For this review, take the finished solid that the model builds, in its own axes (mm). Face numbers are marked on the shaded views. Round coordinates to 2 decimals unless told otherwise and drop trailing zeros. Order: outer loops, then holes, each group sorted by start corner. A loop starts at its lowest first (then second) coordinate and runs counter-clockwise, first axis right, second up. Notation, with made-up numbers: M -35,55.25 L -18,55.25 A17 ccw -18,73.25 Z; hole C 10.5,-13.75 d5. An arc over 180 degrees is marked long. Use a Markdown table: item, result.
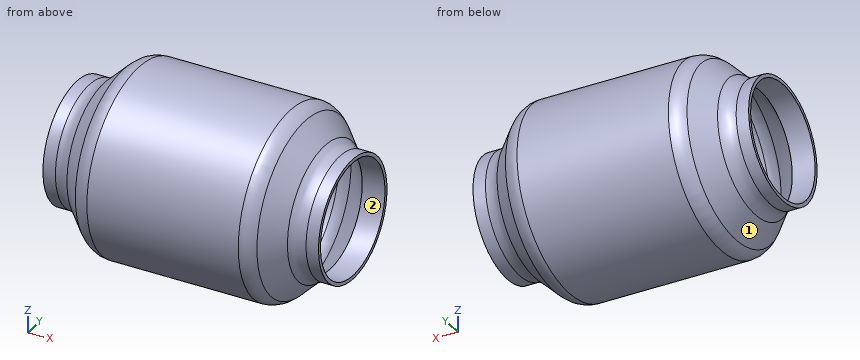
from build123d import *


with BuildPart() as part:
    # Sketch1 → Revolve1 (revolve)
    with BuildSketch(Plane.XY):
        with BuildLine():
            Line((-123.19, 53.975), (-123.19, 50.8))
            Line((-123.19, 50.8), (-102.824871939, 50.8))
            Line((-102.824871939, 50.8), (-79.829487758, 73.795384182))
            ThreePointArc((-79.829487758, 73.795384182), (-73.649222963, 77.924905094), (-66.359103576, 79.375))
            Line((-66.359103576, 79.375), (66.359103576, 79.375))
            ThreePointArc((66.359103576, 79.375), (73.649222963, 77.924905094), (79.829487758, 73.795384182))
            Line((79.829487758, 73.795384182), (102.824871939, 50.8))
            Line((102.824871939, 50.8), (123.19, 50.8))
            Line((123.19, 50.8), (123.19, 53.975))
            Line((123.19, 53.975), (112.030768363, 53.975))
            ThreePointArc((112.030768363, 53.975), (104.740648977, 55.425094906), (98.560384182, 59.554615818))
            Line((98.560384182, 59.554615818), (81.144615818, 76.970384182))
            ThreePointArc((81.144615818, 76.970384182), (74.964351023, 81.099905094), (67.674231637, 82.55))
            Line((67.674231637, 82.55), (-67.674231637, 82.55))
            ThreePointArc((-67.674231637, 82.55), (-74.964351023, 81.099905094), (-81.144615818, 76.970384182))
            Line((-81.144615818, 76.970384182), (-98.560384182, 59.554615818))
            ThreePointArc((-98.560384182, 59.554615818), (-104.740648977, 55.425094906), (-112.030768363, 53.975))
            Line((-112.030768363, 53.975), (-123.19, 53.975))
        make_face()
    revolve(axis=Axis((-123.19, 0, 0), (1, 0, 0)))


solid = part.part
Q1. Add section A-A (x = 11). Write out the cut boundary in (y, z) (3 decimals), then the cut area to 3 significant figures.
Determined:
| item | result |
|---|---|
| outline | C 0,0 d165.1; hole C 0,0 d158.75 |
| area | 1,620 mm^2 |
Q2. Wall thickness on line 1 along Z through (x, y) = (-27, 0) (3 decimals); line 2 along X through (y, z) = (12.5, 58.5); line 3 along Y through (x, z) = (-89, 15.5): over which ranges is each line inside the solid? List them lowest first. Write a range as [from, to].
Determined:
| item | result |
|---|---|
| line 1 | z = [-82.55, -79.375], [79.375, 82.55] |
| line 2 | x = [-98.29, -93.8], [93.8, 98.29] |
| line 3 | y = [-67.35, -62.74], [62.74, 67.35] |
Q3. Draft analysis for pull direction Y (two halves, no side actions). For the marked faces 1 and 2, state which applies: pulls with the +Y half, pulls with the -Y half, needs draft (parallel to the pull), parting line crosses it, or undercut.
Determined:
| item | result |
|---|---|
| face 1 | parting line crosses it |
| face 2 | undercut |
Q4. Clearance check with flat-ended pins moving along their axes: pin 1 (1 mm diameter, centred on x = -54, y = 58, fed in from +Z); pin 2 (8 mm diameter, centred on x = -3, z = -11.5, fed in from +Y); pin 3 (8 mm diameter, centred on x = 18, z = 14, fed in from +Y). State where each tip first meets the part, or that it passes through.
Determined:
| item | result |
|---|---|
| pin 1 | stops at z = 59.23 |
| pin 2 | stops at y = 82.21 |
| pin 3 | stops at y = 81.94 |
Q5. Add section B-B (x = 89.5). Write out the cut boundary in (y, z) (3 decimals), then the cut area to 3 significant figures.
Determined:
| item | result |
|---|---|
| outline | C 0,0 d137.23; hole C 0,0 d128.25 |
| area | 1,870 mm^2 |
